The listing builds one solid part. Answer for the finished solid, in the listing's coordinates (mm). A direction names the side the tool comes from. Give positions to 0.01 mm unless a question says otherwise; leave off trailing zeros. Write each loop counter-clockwise with the first axis right and the second up, starting at its lowest first coordinate (ties: lowest second). Pieces come first, ordered by that corner, then holes. Notation, with made-up numbers: (-3.5, -1.5) - (41.5, -1.5) arc R6 cw to (41.5, 8.5) - close; hole circle Ø7 at (48, 10). An arc over 180 degrees is marked (long way). One line per question, with ' | ' between items. Start each with the question number.
1. A cutting plane is placed at A-A (x = 9). Determine the outline of the cut face in (y, z), then the cut area to 3 significant figures.
2. For faces 4 (the face through (-13, 1, 13.5)), 5 (the face through (10, 1, -15)), 6 (the face through (12, 1, 13.5)), 7 (the face through (-10, 1, -15)), 8 (the face through (-10, 2, 9)), determine the directions among +Z, -Z, +X, -X, +Y, -Y from which every point of the face is accessible in a straight line to the end or side of a thin tool.
3. The mould has two halves that part along X. Classify faces 1 (the face through (10, 2, 9)), 2 (the face through (0, 1, 16)), 3 (the face through (-10, 1, 15)): +X half, -X half, draft (parallel to the pull), parting line (faces both ways), or undercut.
4. Find the intervals of material crossed by L1, parallel to Z at x = -4.5, y = 2.95; L2, parallel to X at y = 2.7, z = 9.5; L3, parallel to Z at x = 11.25, y = 1.5, in increasing order. Write a range as from..to.
5. Given P1, Ø1.2, axis at y = 1.5, z = -15, coming from the +X side; P2, Ø4, axis at x = 8, z = -5, coming from the -Y side, each flat-ended and moving along its own axis, determine where each tip first touches the part or whether it passes through.
6. A cutting plane is placed at B-B (y = 2). Determine the outline of the cut face in (x, z), then the cut area to 3 significant figures.
```python
from build123d import *

# Parameters (mm, degrees)
SKETCH_1_W          = 20
SKETCH_1_H          = 2.5
SKETCH_1_W_2        = 30
SKETCH_1_H_2        = 27
EXTRUDE_1_DEPTH     = 3
SKETCH_2_W          = 20
SKETCH_2_H          = 3
CUT_EXTRUDE_1_DEPTH = 23.135943621


with BuildPart() as part:
    # 草图1 → 凸台-拉伸1 (new body)
    with BuildSketch(Plane(origin=(0, 0, 0), x_dir=(1, 0, 0), z_dir=(0, 1, 0))):
        with Locations((0, 14.75)):
            Rectangle(SKETCH_1_W, SKETCH_1_H)
        Rectangle(SKETCH_1_W_2, SKETCH_1_H_2)
        with Locations((0, -14.75)):
            Rectangle(SKETCH_1_W, SKETCH_1_H)
    extrude(amount=EXTRUDE_1_DEPTH)

    # 草图2 → 切除-拉伸1 (cut, through all)
    with BuildSketch(Plane(origin=(0, 3, 0), x_dir=(1, 0, 0), z_dir=(0, 1, 0))):
        with Locations((0, -9)):
            Rectangle(SKETCH_2_W, SKETCH_2_H)
        with Locations((0, -3)):
            Rectangle(SKETCH_2_W, SKETCH_2_H)
    extrude(amount=-CUT_EXTRUDE_1_DEPTH, mode=Mode.SUBTRACT)


solid = part.part
```
Determined:
1) outline: (0, -16) - (3, -16) - (3, 1.5) - (0, 1.5) - close; (0, 4.5) - (3, 4.5) - (3, 7.5) - (0, 7.5) - close; (0, 10.5) - (3, 10.5) - (3, 16) - (0, 16) - close | area: 78.0 mm2
2) face 4: +Z, -X, +Y, -Y | face 5: -Z, +X, +Y, -Y | face 6: +Z, +X, +Y, -Y | face 7: -Z, -X, +Y, -Y | face 8: +Y, -Y
3) face 1: undercut | face 2: draft | face 3: -X half
4) L1: -16..1.5, 4.5..7.5, 10.5..16 | L2: -15..-10, 10..15 | L3: -13.5..13.5
5) P1: x = 10 | P2: y = 0
6) outline: (-15, -13.5) - (-10, -13.5) - (-10, -16) - (10, -16) - (10, -13.5) - (15, -13.5) - (15, 13.5) - (10, 13.5) - (10, 16) - (-10, 16) - (-10, 13.5) - (-15, 13.5) - close; hole (-10, 1.5) - (10, 1.5) - (10, 4.5) - (-10, 4.5) - close; hole (-10, 7.5) - (10, 7.5) - (10, 10.5) - (-10, 10.5) - close | area: 790 mm2
